Build history of the part. All positions in model axes, mm. Face numbers are marked on the shaded views. A direction names the side the tool comes from. Give positions to 0.01 mm unless a question says otherwise; leave off trailing zeros. Write each loop counter-clockwise with the first axis right and the second up, starting at its lowest first coordinate (ties: lowest second). Pieces come first, ordered by that corner, then holes. Notation, with made-up numbers: (-4, 76.25) -> (30, 76.25) arc R29 ccw to (30, 104.25) -> close; hole circle Ø11 at (10, 15.5). An arc over 180 degrees is marked (long way). Put each result on its own line as item: value.
Autodesk Inventor part; units mm, degrees
ref_plane "YZ Plane" through (0, 0, 0) normal (1, 0, 0) x (0, 1, 0)
ref_plane "XZ Plane" through (0, 0, 0) normal (0, 1, 0) x (-1, 0, 0)
ref_plane "XY Plane" through (0, 0, 0) normal (0, 0, 1) x (1, 0, 0)
sketch "Sketch1" plane through (0, 0, 0) normal (0, 0, 1) x (1, 0, 0)
  line L0 (-4, 4) -> (4, 4)
  line L1 (4, 4) -> (4, -4)
  line L2 (4, -4) -> (-4, -4)
  line L3 (-4, -4) -> (-4, 4)
  line L4 (-4, -4) -> (4, 4) construction
  point P0 (0, 0)
  point P1 (0, 0)
  dimension "d0" = 8
extrude "Extrusion1" add sketch "Sketch1" along normal blind 4
sketch "Sketch2" plane through (0, 0, 4) normal (0, 0, 1) x (1, 0, 0)
  circle A0 centre (0, 0) radius 3
  dimension "d3" = 6
extrude "Extrusion2" add sketch "Sketch2" along normal blind 0.7
sketch "Sketch3" plane through (0, 0, 4.7) normal (0, 0, 1) x (1, 0, 0)
  circle A0 centre (0, 0) radius 2
  dimension "d6" = 4
extrude "Extrusion3" add sketch "Sketch3" along normal blind 6
properties part number "Arm - forearm v2 3"
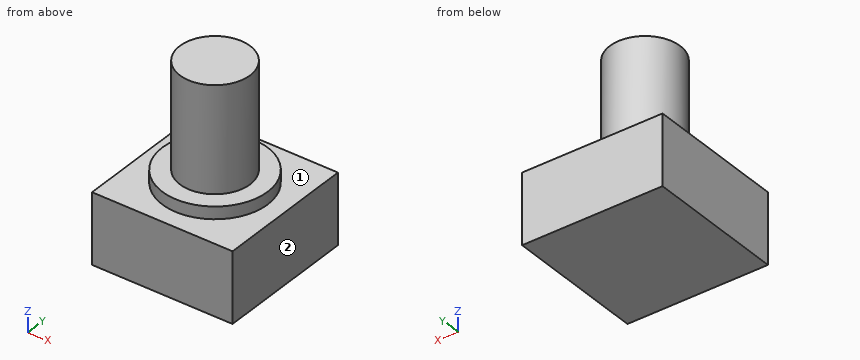
1) Wall check: L1, parallel to Z at x = 1.75, y = -1.5; L2, parallel to Z at x = -0.5, y = 3.75; L3, parallel to X at y = -0.5, z = 5. Give the ranges that are in metal, low to high.
Filled sheet:
L1: 0 to 4.7
L2: 0 to 4
L3: -1.94 to 1.94
2) Slice it at D-D (y = 2.5). Write the cut outline in (x, z).
Filled sheet:
outline: (-4, 0) -> (4, 0) -> (4, 4) -> (1.66, 4) -> (1.66, 4.7) -> (-1.66, 4.7) -> (-1.66, 4) -> (-4, 4) -> close
3) Tool access for the marked faces 1 and 2: list every direction of +Z, -Z, +X, -X, +Y, -Y with a clear straight run to the whole face (end or side of a thin tool).
Filled sheet:
face 1: +Z
face 2: +Z, -Z, +X, +Y, -Y
4) Slice it at A-A (x = 0). Write the cut outline in (y, z).
Filled sheet:
outline: (-4, 0) -> (4, 0) -> (4, 4) -> (3, 4) -> (3, 4.7) -> (2, 4.7) -> (2, 10.7) -> (-2, 10.7) -> (-2, 4.7) -> (-3, 4.7) -> (-3, 4) -> (-4, 4) -> close
5) Slice it at C-C (z = 9). Write the cut outline in (x, y).
Filled sheet:
outline: circle Ø4 at (0, 0)
6) Pin check, flat tips, straight feed: pin 1 (1.5 mm diameter, centred on y = -1.5, z = 9.5, fed in from -X); pin 2 (2 mm diameter, centred on x = -3, y = 2.5, fed in from +Z). Stop position of each tip, or through.
Filled sheet:
pin 1: x = -1.85
pin 2: z = 4.7
